Verification items for the finished model (mm, model axes). Face numbers are marked on the shaded views. A direction names the side the tool comes from. Round coordinates to 2 decimals unless told otherwise and drop trailing zeros. Write each loop counter-clockwise with the first axis right and the second up, starting at its lowest first coordinate (ties: lowest second). Pieces come first, ordered by that corner, then holes. Notation, with made-up numbers: (-22.5, -3.75) - (6.5, -3.75) arc R37 ccw to (6.5, 33.25) - close; hole circle Ø4 at (27, -27). An arc over 180 degrees is marked (long way). Write each question's results on one line, items separated by ' | '.
```python
from build123d import *


with BuildPart() as part:
    # Sketch1 → Revolve1 (revolve)
    with BuildSketch(Plane.XY, mode=Mode.PRIVATE) as revolve1_sk:
        with BuildLine():
            Line((12, 24.5), (12, 21.591227021))
            Line((12, 21.591227021), (16.182938488, 21.591227021))
            Line((16.182938488, 21.591227021), (16.182938488, 17.471972716))
            Line((16.182938488, 17.471972716), (28.817061512, 17.471972716))
            Line((28.817061512, 17.471972716), (28.817061512, 21.591227021))
            Line((28.817061512, 21.591227021), (33.001856356, 21.591227021))
            Line((33.001856356, 21.591227021), (33.001856356, 24.5))
            Line((33.001856356, 24.5), (33, 24.5))
            Line((33, 24.5), (27.817061512, 24.5))
            Line((27.817061512, 24.5), (24.746847829, 24.753346743))
            Line((24.746847829, 24.753346743), (23.272118433, 24.875037911))
            ThreePointArc((23.272118433, 24.875037911), (22.5, 25.299429712), (21.727881567, 24.875037911))
            Line((21.727881567, 24.875037911), (20.253152171, 24.753346743))
            Line((20.253152171, 24.753346743), (17.182938488, 24.5))
            Line((17.182938488, 24.5), (12, 24.5))
        make_face()
    revolve(revolve1_sk.sketch.rotate(Axis((0, 0, 0), (1, 0, 0)), 90), axis=Axis((0, 0, 0), (1, 0, 0)))


solid = part.part
```
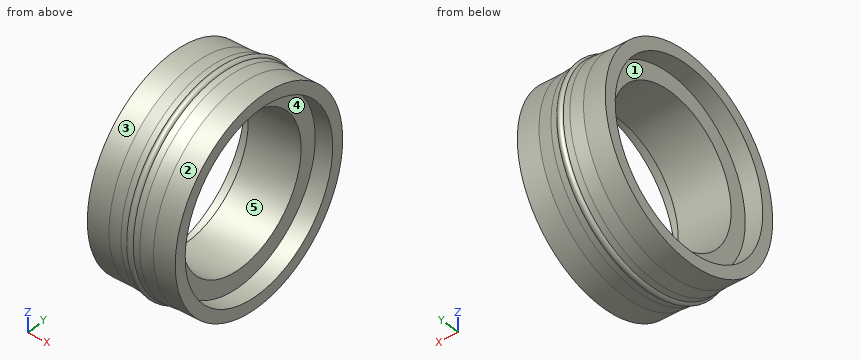
(1) Section check B-B (x = 26.25). Record the cut outline in (y, z).
Answer:
outline: circle Ø49.26 at (0, 0); hole circle Ø34.94 at (0, 0)
(2) Thickness scan on L1, parallel to Y at x = 15, z = 0.5; L2, parallel to Y at x = 25.5, z = -4; L3, parallel to X at y = 16.5, z = 7.5. Record the ranges inside material, lowest first.
Answer:
L1: -24.49 to -21.59, 21.59 to 24.49 | L2: -24.37 to -17.01, 17.01 to 24.37 | L3: 16.18 to 28.82
(3) Set-up check for the marked faces 1 and 2: record each of +Z, -Z, +X, -X, +Y, -Y from which the full face is reachable in a straight line by a thin tool's end or side.
Answer:
face 1: -X | face 2: +X
(4) Go/stop test with flat-tipped pins: pin 1 Ø3 at (x, z) = (18, 2.5) entering from -Y; pin 2 Ø21.5 at (y, z) = (-2.5, -9) entering from +X; pin 3 Ø2 at (x, z) = (22, -1) entering from +Y. Record where each tip stops, or that it passes through.
Answer:
pin 1: y = -24.61 | pin 2: x = 28.82 | pin 3: y = 25.3
(5) Section check A-A (x = 19). Record the cut outline in (y, z), plus the area to 3 significant figures.
Answer:
outline: circle Ø49.3 at (0, 0); hole circle Ø34.94 at (0, 0) | area: 950 mm2
(6) Mould release check, pull along Y, two halves, no side actions. Record for the marked faces 3, 4 and 5: released by +Y, released by -Y, zero draft, split by the parting line, or undercut.
Answer:
face 3: split by the parting line | face 4: undercut | face 5: undercut
